Geometry: final body of the model. Coordinates: model frame, mm. A direction names the side the tool comes from. Coordinates: 2 decimals unless noted, no trailing zeros. Write each loop counter-clockwise with the first axis right and the second up, starting at its lowest first coordinate (ties: lowest second). Pieces come first, ordered by that corner, then holes. Notation, with made-up numbers: (-8.5, -16.75) -> (37.5, -16.75) arc R15 ccw to (37.5, -4.75) -> close; hole circle Ø7 at (32.5, 53). An arc over 180 degrees is marked (long way). One line per item, written item: value. Start each with the question number.
from build123d import *

# Parameters (mm, degrees)
F0_W          = 116.84
F0_H          = 76.2
F1_DEPTH      = 101.6
F3_DEPTH      = 76.2
F5_DEPTH      = 38.1
F5_DEPTH_BACK = 38.1
F6_R          = 3.1115
F7_DEPTH      = 114.3
F7_DEPTH_BACK = 114.3
F9_DEPTH      = 101.601
F11_DEPTH     = 25.401
F12_SIZE      = 5.08
F13_W         = 177.8
F13_H         = 62.1990481529
F14_DEPTH     = 76.2
F15_W         = 93.98
F15_H         = 7.62
F16_DEPTH     = 25.4
F18_DEPTH     = 7.62
F20_DEPTH     = 7.62
F21_R         = 3.175
F22_DEPTH     = 6.35
F23_DEPTH     = 19.05


with BuildPart() as f1:
    # F0 (on Front) → F1 (new body)
    with BuildSketch(Plane.XZ):
        with Locations((58.42, 38.1)):
            Rectangle(F0_W, F0_H)
        with Locations((-58.42, 38.1)):
            Rectangle(F0_W, F0_H)
        with Locations((58.42, -38.1)):
            Rectangle(F0_W, F0_H)
        with Locations((-58.42, -38.1)):
            Rectangle(F0_W, F0_H)
    extrude(amount=-F1_DEPTH)

    # F2 (on face) → F3 (cut)
    with BuildSketch(Plane.XZ):
        Polygon((-38.1, -12.7), (-104.14, -12.7), (-104.14, -69.85), (-104.14, -76.2), (104.14, -76.2), (104.14, -69.85), (104.14, -12.7), (38.1, -12.7), (38.1, 63.5), (-38.1, 63.5), align=None)
    extrude(amount=-F3_DEPTH, mode=Mode.SUBTRACT)

    # F4 (on Right) → F5 (cut, two sides)
    with BuildSketch(Plane.YZ) as f5_sk:
        Polygon((0, 71.12), (0, 63.5), (76.2, 63.5), align=None)
    extrude(amount=-F5_DEPTH, mode=Mode.SUBTRACT)
    extrude(f5_sk.sketch, amount=F5_DEPTH_BACK, mode=Mode.SUBTRACT)

    # F6 (on Right) → F7 (join, two sides)
    with BuildSketch(Plane.YZ) as f7_sk:
        with BuildLine():
            ThreePointArc((25.4005372305, 50.8), (29.8906652911, 52.6598719395), (31.7505372305, 57.15))
            ThreePointArc((31.7505372305, 57.15), (20.91040917, 61.6401280605), (25.4005372305, 50.8))
        make_face()
        with Locations((50.8005372305, -41.021)):
            Circle(F6_R)
        with Locations((50.8005372305, -61.087)):
            Circle(F6_R)
    extrude(amount=F7_DEPTH)
    extrude(f7_sk.sketch, amount=-F7_DEPTH_BACK)

    # F8 (on face) → F9 (cut, through all)
    with BuildSketch(Plane.XZ):
        with BuildLine():
            Line((-46.99, 76.2), (-116.84, 76.2))
            Line((-116.84, 76.2), (-116.84, 0))
            Line((-116.84, 0), (-97.79, 0))
            ThreePointArc((-97.79, 0), (-61.8689755157, 14.8789755157), (-46.99, 50.8))
            Line((-46.99, 50.8), (-46.99, 76.2))
        make_face()
        with BuildLine():
            Line((116.84, 0), (116.84, 76.2))
            Line((116.84, 76.2), (46.99, 76.2))
            Line((46.99, 76.2), (46.99, 50.8))
            ThreePointArc((46.99, 50.8), (61.8689755157, 14.8789755157), (97.79, 0))
            Line((97.79, 0), (116.84, 0))
        make_face()
    extrude(amount=-F9_DEPTH, mode=Mode.SUBTRACT)

    # F10 (on face) → F11 (cut, through all)
    with BuildSketch(Plane.XZ.offset(-76.2)):
        Polygon((104.14, -76.2), (104.14, -48.7679988146), (104.14, -46.2279988146), (-104.14, -46.2279988146), (-104.14, -48.7679988146), (-104.14, -76.2), align=None)
    extrude(amount=-F11_DEPTH, mode=Mode.SUBTRACT)

    # F12
    f12_edges = [f1.edges().sort_by_distance(p)[0] for p in [
        (104.14, 50.8, -76.2),
        (-104.14, 50.8, -76.2),
    ]]
    chamfer(f12_edges, length=F12_SIZE)

    # F13 (on Front) → F14 (cut)
    with BuildSketch(Plane.XZ):
        with Locations((0, -55.8045858206)):
            Rectangle(F13_W, F13_H)
    extrude(amount=-F14_DEPTH, mode=Mode.SUBTRACT)

    # F15 (on face) → F16 (join)
    with BuildSketch(Plane.XY.offset(76.2)):
        with Locations((0, 97.79)):
            Rectangle(F15_W, F15_H)
    extrude(amount=F16_DEPTH)

    # F17 (on face) → F18 (join)
    with BuildSketch(Plane.YZ.offset(46.99)):
        Polygon((93.98, 76.2), (93.98, 101.6), (30.48, 76.2), align=None)
    extrude(amount=-F18_DEPTH)

    # F19 (on face) → F20 (join)
    with BuildSketch(Plane(origin=(-46.99, 0, 0), x_dir=(0, -1, 0), z_dir=(-1, 0, 0))):
        Polygon((-30.48, 76.2), (-93.98, 101.6), (-93.98, 76.2), align=None)
    extrude(amount=-F20_DEPTH)

    # F21 (on face) → F22 (join)
    with BuildSketch(Plane.YZ.offset(-104.14)):
        with BuildLine():
            Line((6.0337829095, -9.5307531462), (-1.0780708533, -11.3087165869))
            Line((-1.0780708533, -11.3087165869), (-102.6780708533, -36.7087165869))
            ThreePointArc((-102.6780708533, -36.7087165869), (-105.9122834131, -42.0990708533), (-100.5219291467, -45.3332834131))
            Line((-100.5219291467, -45.3332834131), (0, -20.2028011265))
            Line((0, -20.2028011265), (1.0780708533, -19.9332834131))
            Line((1.0780708533, -19.9332834131), (14.6432286128, -19.9332834131))
            Line((14.6432286128, -19.9332834131), (14.6432286128, -9.5307531462))
            Line((14.6432286128, -9.5307531462), (6.0337829095, -9.5307531462))
        make_face()
        with Locations((-101.6, -41.021)):
            Circle(F21_R, mode=Mode.SUBTRACT)
        with Locations((-101.6, -41.021)):
            Circle(F21_R)
    extrude(amount=F22_DEPTH)

    # F21 (on face) → F23 (join)
    with BuildSketch(Plane.YZ.offset(-104.14)):
        with Locations((-101.6, -41.021)):
            Circle(F21_R)
    extrude(amount=F23_DEPTH)

    # F24: F1 across plane


with BuildPart() as f1_1:
    add(f1.part)
    add(f1.part.mirror(Plane.YZ))


solid = f1_1.part
Q1. Access query for faces 1 (the flat face through (-39.37, 77, 83)), 2 (the cylindrical face through (-96.627, 47.692, -60.95)), 3 (the flat face through (88.9, 51, -61)), 4 (the flat face through (-101, 8, -19.933)), 5 (the flat face through (-107, 50, 0)). Directions: +Z, -Z, +X, -X, +Y, -Y. A direction counts if a zero-diameter tool reaches every point of the face in a straight line with its end or side. Return the directions, or none.
Q2. Cut plane B-B on z = 90. Output: boundary loops of the cut face in (x, y), and give its area (3 significant figures).
Q3. First-contact query: P1, Ø12.5, axis at x = 3, z = 92.5, coming from the -Y side; P2, Ø12, axis at y = 46, z = 49, coming from the -X side; P3, Ø2, axis at x = 35, z = 72, coming from the -Y side. Flat tips, straight axial feed; report the tip coordinate or a pass-through.
Q4. Draft query along Y for faces 6 (the flat face through (104.14, 39, -42)), 7 (the flat face through (-116.84, 50, -38)), 8 (the flat face through (-44, 0, 6)). Return one class per face: pulls with the +Y half, pulls with the -Y half, needs draft (parallel to the pull), parting line crosses it, or undercut.
Q5. Cut plane D-D on x = -53.5. Output: boundary loops of the cut face in (y, z).
Q6. Cut plane A-A on x = -13. Output: boundary loops of the cut face in (y, z), and give its area (3 significant figures).
Q7. Cut plane C-C on y = -57. Output: boundary loops of the cut face in (x, z), and give its area (3 significant figures).
Q8. Line query: L1, parallel to X at y = 36.5, z = 77; L2, parallel to X at y = 61, z = 54.5; L3, parallel to Z at x = -38.5, y = 83. Output: solid intervals per line, ascending. Write a range as from..to.
Solution:
1. face 1: +Z, -Y
1. face 2: none
1. face 3: -Z, +Y, -Y
1. face 4: -Z
1. face 5: +Z, -X, +Y, -Y
2. outline: (-46.99, 64.98) -> (-39.37, 64.98) -> (-39.37, 93.98) -> (39.37, 93.98) -> (39.37, 64.98) -> (46.99, 64.98) -> (46.99, 101.6) -> (-46.99, 101.6) -> close
2. area: 1,160 mm²
3. P1: y = 93.98
3. P2: x = -47.59
3. P3: y = 0
4. face 6: undercut
4. face 7: needs draft
4. face 8: pulls with the -Y half
5. outline: (0, -12.7) -> (76.2, -12.7) -> (76.2, -46.23) -> (101.6, -46.23) -> (101.6, 25.92) -> (0, 25.92) -> close
6. outline: (0, 71.12) -> (76.2, 63.5) -> (76.2, -46.23) -> (101.6, -46.23) -> (101.6, 101.6) -> (93.98, 101.6) -> (93.98, 76.2) -> (0, 76.2) -> close; circle Ø12.7 at (25.4, 57.15)
6. area: 4,110 mm²
7. outline: (-104.14, -34.45) -> (-97.79, -34.45) -> (-97.79, -25.29) -> (-104.14, -25.29) -> close; (97.79, -34.45) -> (104.14, -34.45) -> (104.14, -25.29) -> (97.79, -25.29) -> close
7. area: 116 mm²
8. L1: -46.99..-39.37, 39.37..46.99
8. L2: -46.99..-38.1, 38.1..46.99
8. L3: -46.23..76.2
